Autodesk Inventor part; units mm, degrees
ref_plane "YZ Plane" through (0, 0, 0) normal (1, 0, 0) x (0, 1, 0)
ref_plane "XZ Plane" through (0, 0, 0) normal (0, 1, 0) x (-1, 0, 0)
ref_plane "XY Plane" through (0, 0, 0) normal (0, 0, 1) x (1, 0, 0)
sketch "Sketch1" plane through (0, 0, 0) normal (0, 0, 1) x (1, 0, 0)
  line L0 (-2.5, -35.0001) -> (2.5, -35.0001)
  line L1 (2.8921, 7.4595) -> (4.1309, 9.1069)
  line L2 (-2.8882, 7.4611) -> (-3.0825, 9.5131)
  line L3 (-3.0825, 9.5131) -> (-5.3884, 5.9139)
  line L4 (-5.3884, 5.9139) -> (-6.3108, 7.7572)
  line L5 (-6.3108, 7.7572) -> (-7.1609, 3.5681)
  line L6 (-7.1609, 3.5681) -> (-8.6869, 4.9536)
  line L7 (-8.6869, 4.9536) -> (-7.9662, 0.7403)
  line L8 (-7.9662, 0.7403) -> (-9.8897, 1.481)
  line L9 (-9.8897, 1.481) -> (-7.6957, -2.1874)
  line L10 (-7.6957, -2.1874) -> (-9.7569, -2.1916)
  line L11 (-9.7569, -2.1916) -> (-6.3859, -4.8197)
  line L12 (-6.3859, -4.8197) -> (-8.3064, -5.5682)
  line L13 (-8.3064, -5.5682) -> (-4.2136, -6.8011)
  line L14 (-4.2136, -6.8011) -> (-5.734, -8.1928)
  line L15 (-5.734, -8.1928) -> (-1.4722, -7.864)
  line L16 (-1.4722, -7.864) -> (-2.3872, -9.7109)
  line L17 (-2.3872, -9.7109) -> (1.468, -7.8647)
  line L18 (1.468, -7.8647) -> (1.282, -9.9175)
  line L19 (1.282, -9.9175) -> (4.21, -6.8033)
  line L20 (4.21, -6.8033) -> (4.778, -8.7847)
  line L21 (4.778, -8.7847) -> (6.3833, -4.8231)
  line L22 (6.3833, -4.8231) -> (7.6287, -6.4655)
  line L23 (7.6287, -6.4655) -> (7.6946, -2.1915)
  line L24 (7.6946, -2.1915) -> (9.4492, -3.273)
  line L25 (9.4492, -3.273) -> (7.9666, 0.7361)
  line L26 (7.9666, 0.7361) -> (9.9935, 0.3614)
  line L27 (9.9935, 0.3614) -> (7.1628, 3.5643)
  line L28 (7.1628, 3.5643) -> (9.1881, 3.9471)
  line L29 (9.1881, 3.9471) -> (5.3915, 5.9111)
  line L30 (5.3915, 5.9111) -> (7.1418, 6.9996)
  line L31 (7.1418, 6.9996) -> (2.8921, 7.4595)
  line L32 (-2.5, -35) -> (2.5, -35)
  line L33 (2.5, 35) -> (-2.5, 35)
  arc A0 (-2.5, -7.011) -> (2.5, -7.011) centre (0, 0) ccw
  line L34 (2.5, -7.011) -> (2.5, 35)
  line L35 (-2.5, 35) -> (-2.5, -7.011)
  circle A1 centre (0, 16) radius 0.75
  circle A2 centre (0, 0) radius 0.75
  dimension "d3" = 5
  dimension "d5" = 1.5
  dimension "d6" = 1.5
extrude "Extrusion1" add sketch "Sketch1" along normal blind 2
sketch "Sketch2" plane through (0, 0, 2) normal (0, 0, 1) x (1, 0, 0)
  circle A0 centre (0, 0) radius 0.75
  line L0 (2.5, 18) -> (2.5, 35)
  line L1 (2.5, 35) -> (-2.5, 35)
  line L2 (-2.5, 35) -> (-2.5, 18)
  line L3 (2.5, 18) -> (-2.5, 18)
  line L4 (-2.5, 35) -> (-2.5, -7.011)
extrude "Extrusion2" add sketch "Sketch2" along normal blind 11 contours L3 L2 L1 L0
properties part number "Valve"
CAD build for the part. Positions are in the model's coordinates, mm. A direction names the side the tool comes from. Round coordinates to 2 decimals unless told otherwise and drop trailing zeros. Write each loop counter-clockwise with the first axis right and the second up, starting at its lowest first coordinate (ties: lowest second). Pieces come first, ordered by that corner, then holes. Notation, with made-up numbers: (48, 63) - (68, 63) arc R27 cw to (68, 84) - close; hole circle Ø2 at (-14.5, 87.5). An arc over 180 degrees is marked (long way). Return JSON: item names as keys, results as strings. Group by question number.
Item 1: 3-axis set-ups, long thin cutter, end or side, ignore diameter. For faces 5 (the face through (0, 27, 13)), 6 (the face through (0, 5, 2)): which of +Z, -Z, +X, -X, +Y, -Y reach the whole face in a straight line?
Item 2: Band-saw the part on B-B on y = 0. List the corners of the cut face in (x, z), plus the area to 3 significant figures.
Item 3: Mould opens along X. For faces 1 (the face through (0.036, -7.443, 0.986)), 2 (the face through (0, 18, 7)), 3 (the face through (-0.595, 16.456, 0.986)), 4 (the face through (-0.75, -0.03, 0.99)) say: +X half, -X half, draft (parallel to the pull), parting line (faces both ways), or undercut.
Item 4: Band-saw the part on A-A on x = 0. List the corners of the cut face in (y, z), plus the area to 3 significant figures.
Item 5: Band-saw the part on C-C on z = 8.5. List the corners of the cut face in (x, y).
Item 6: Flat gauge pins, fed straight in: pin 1 Ø4 at (y, z) = (2, 5) entering from -X; pin 2 Ø2 at (x, y) = (-1, 6.5) entering from +Z; pin 3 Ø1 at (x, z) = (0, 3) entering from -Y. Where does each tip first touch, or does it go through?
Item 7: Probe probe 1 along Y at (x, z) = (0, 0.9); probe 2 along Y at (x, z) = (1.7, 6.75); probe 3 along Z at (x, y) = (-2.3, -4). List the from-to ranges inside material, lowest first.
Resolved:
{
 "1": {"face 5": "+Z, +X, -X, +Y, -Y", "face 6": "+Z, +X, -X, -Y"},
 "2": {"outline": "(-2.5, 0) - (-0.75, 0) - (-0.75, 2) - (-2.5, 2) - close; (0.75, 0) - (2.5, 0) - (2.5, 2) - (0.75, 2) - close", "area": "7.00 mm²"},
 "3": {"face 1": "parting line", "face 2": "draft", "face 3": "undercut", "face 4": "undercut"},
 "4": {"outline": "(-7.44, 0) - (-0.75, 0) - (-0.75, 2) - (-7.44, 2) - close; (0.75, 0) - (15.25, 0) - (15.25, 2) - (0.75, 2) - close; (16.75, 0) - (35, 0) - (35, 13) - (18, 13) - (18, 2) - (16.75, 2) - close", "area": "266 mm²"},
 "5": {"outline": "(-2.5, 18) - (2.5, 18) - (2.5, 35) - (-2.5, 35) - close"},
 "6": {"pin 1": "passes through", "pin 2": "stops at z = 2", "pin 3": "stops at y = 18"},
 "7": {"probe 1": "y = -7.44 to -0.75, 0.75 to 15.25, 16.75 to 35", "probe 2": "y = 18 to 35", "probe 3": "z = 0 to 2"}
}
